Geometry check sheet. Reference: the model listing, model coordinates, mm. Face numbers are marked on the shaded views. A direction names the side the tool comes from. Give positions to 0.01 mm unless a question says otherwise; leave off trailing zeros. Write each loop counter-clockwise with the first axis right and the second up, starting at its lowest first coordinate (ties: lowest second). Pieces come first, ordered by that corner, then holes. Notation, with made-up numbers: (80, 55) - (90, 55) arc R20 cw to (90, 82) - close; hole circle Ø3 at (-9, 65.25). An arc over 180 degrees is marked (long way). One line per question, with ' | ' between items. Start each with the question number.
Q1. Release check for a two-part mould opening along X. For the marked faces 1, 2 and 3 record: +X half, -X half, draft (parallel to the pull), parting line (faces both ways), or undercut.
Q2. Section check A-A on x = 0. Record the boundary of the cut face in (y, z).
Q3. Section check D-D on x = -10.5. Record the boundary of the cut face in (y, z), and give its area (3 significant figures).
Q4. Set-up check for the marked faces 4, 5 and 6: record each of +Z, -Z, +X, -X, +Y, -Y from which the full face is reachable in a straight line by a thin tool's end or side.
Q5. Gauge pin test, flat ends, axial feed: P1, Ø2, axis at x = 3.5, z = 1.5, coming from the -Y side; P2, Ø3.5, axis at x = 2.5, y = -1.5, coming from the -Z side; P3, Ø6, axis at y = -18.5, z = -1.5, coming from the +X side; P4, Ø2, axis at x = 7, z = 4.5, coming from the -Y side. Record the tip position at first contact, or that the pin passes through.
Q6. Section check C-C on z = -8.5. Record the boundary of the cut face in (x, y), and give its area (3 significant figures).
Q7. Thickness scan on L1, parallel to Y at x = 0, z = -5.75; L2, parallel to Z at x = 11, y = -14.5. Record the ranges inside material, lowest first. Write a range as [from, to].
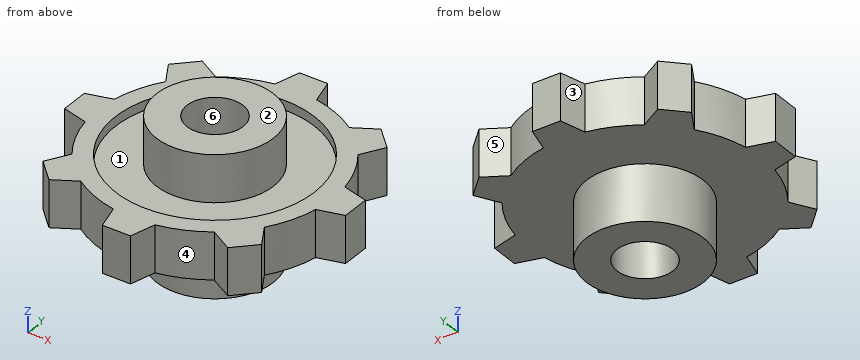
```python
from build123d import *

# Parameters (mm, degrees)
SKETCH1_R           = 25
EXTRUDE1_DEPTH      = 10
EXTRUDE2_DEPTH      = 10
CIRPATTERN1_COUNT   = 8
SKETCH3_R           = 21.25
CUT_EXTRUDE1_DEPTH  = 2
EXTRUDE3_DEPTH      = 10
EXTRUDE3_DEPTH_BACK = 20
SKETCH4_R           = 12.5
SKETCH4_R_2         = 6


with BuildPart() as part:
    # Sketch1 → Extrude1 (new body)
    with BuildSketch(Plane.XY):
        Circle(SKETCH1_R)
    extrude(amount=EXTRUDE1_DEPTH)

    # Sketch2 → Extrude2 (add)
    with BuildSketch(Plane.XY.offset(10)):
        Polygon((-3, 30), (3, 30), (5.679491924, 20), (-5.679491924, 20), align=None)
    extrude2 = extrude(amount=-EXTRUDE2_DEPTH)

    # CirPattern1: Extrude2 ×8 about axis
    cirpattern1_axis = Axis((0, 0, 0), (0, 0, 1))
    for i in range(1, CIRPATTERN1_COUNT):
        add(extrude2.rotate(cirpattern1_axis, i * 360 / CIRPATTERN1_COUNT))

    # Sketch3 → Cut-Extrude1 (cut)
    with BuildSketch(Plane.XY.offset(10)):
        Circle(SKETCH3_R)
    extrude(amount=-CUT_EXTRUDE1_DEPTH, mode=Mode.SUBTRACT)

    # Sketch4 → Extrude3 (add, two sides: drawn at the far end of the back side and taken through both)
    with BuildSketch(Plane.XY.offset(8).offset(-EXTRUDE3_DEPTH_BACK)):
        Circle(SKETCH4_R)
        Circle(SKETCH4_R_2, mode=Mode.SUBTRACT)
    extrude(amount=EXTRUDE3_DEPTH + EXTRUDE3_DEPTH_BACK)


solid = part.part
```
Working result:
1) face 1: undercut | face 2: draft | face 3: -X half
2) outline: (-30, 0) - (-12.5, 0) - (-12.5, -12) - (-6, -12) - (-6, 0) - (6, 0) - (6, -12) - (12.5, -12) - (12.5, 0) - (30, 0) - (30, 10) - (21.25, 10) - (21.25, 8) - (12.5, 8) - (12.5, 18) - (6, 18) - (6, 8) - (-6, 8) - (-6, 18) - (-12.5, 18) - (-12.5, 8) - (-21.25, 8) - (-21.25, 10) - (-30, 10) - close
3) outline: (-22.69, 0) - (-6.78, 0) - (-6.78, -12) - (6.78, -12) - (6.78, 0) - (22.69, 0) - (22.69, 10) - (18.47, 10) - (18.47, 8) - (6.78, 8) - (6.78, 18) - (-6.78, 18) - (-6.78, 8) - (-18.47, 8) - (-18.47, 10) - (-22.69, 10) - close | area: 678 mm2
4) face 4: +Z, -Z, -Y | face 5: +Z, -Z, +Y | face 6: +Z
5) P1: stops at y = -30 | P2: stops at z = 0 | P3: stops at x = 23.33 | P4: stops at y = -24.27
6) outline: circle Ø25 at (0, 0); hole circle Ø12 at (0, 0) | area: 378 mm2
7) L1: y = [-12.5, -6], [6, 12.5] | L2: z = [0, 8]
